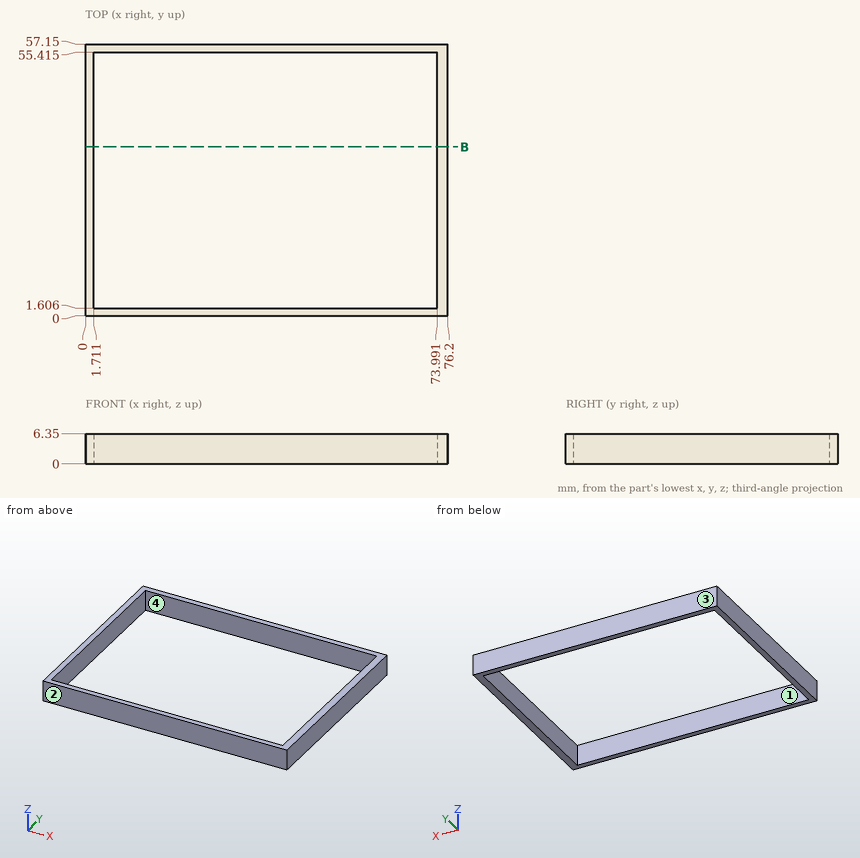
Source: three-view drawing plus pictorial views. Frame: mm from the lowest corner of the part. A direction names the side the tool comes from. Round coordinates to 2 decimals unless told otherwise and drop trailing zeros. Loops run counter-clockwise (first coordinate to the right, second up) from the corner with the lowest first, then second, coordinate; pieces in that order, holes last.
Q1. Pull-direction query (X, two-part tool) for the marked faces 3 and 4; classes: released by +X, released by -X, zero draft, split by the parting line, or undercut.
Q2. Section B-B on y = 35.5. Return loops of the section in (x, z).
Q3. Access query for the marked faces 1 and 2. Directions: +Z, -Z, +X, -X, +Y, -Y. A direction counts if a zero-diameter tool reaches every point of the face in a straight line with its end or side. Return the directions, or none.
Q4. Material intervals for L1, parallel to X at y = 47, z = 2.75, sorted ascending.
Evaluation:
1. face 3: zero draft
1. face 4: undercut
2. outline: (0, 0) - (1.71, 0) - (1.71, 6.35) - (0, 6.35) - close; (73.99, 0) - (76.2, 0) - (76.2, 6.35) - (73.99, 6.35) - close
3. face 1: +Z, -Z
3. face 2: +Z, -Z, +X, -X, -Y
4. L1: x = 0 to 1.71, 73.99 to 76.2
